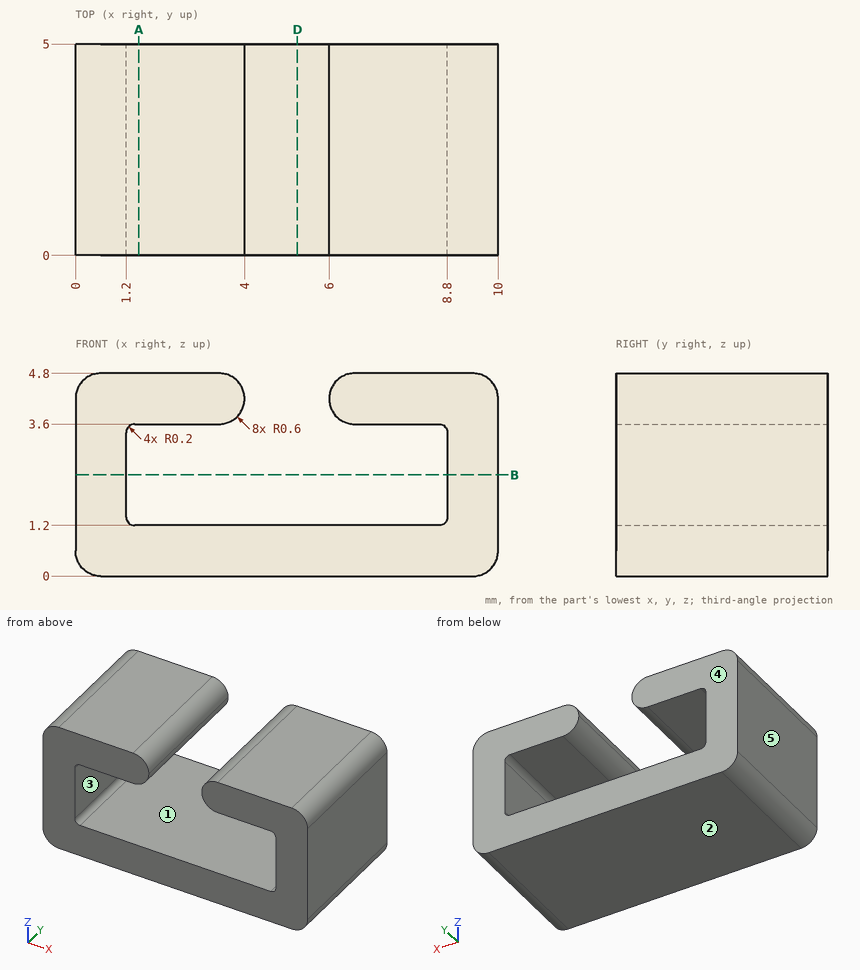
For this review, use the dimensioned drawing (mm, ordinates from the lowest corner) and the shaded views. A direction names the side the tool comes from. Round coordinates to 2 decimals unless told otherwise and drop trailing zeros. Write each loop counter-clockwise with the first axis right and the second up, starting at its lowest first coordinate (ties: lowest second). Pieces come first, ordered by that corner, then holes. Notation, with made-up numbers: (65.25, 46) -> (112.25, 46) arc R24 ccw to (112.25, 57) -> close; hole circle Ø3 at (38, 85). An arc over 180 degrees is marked (long way). Use CSV: the item, a comma, the result in double quotes.
(1) Draft analysis for pull direction X (two halves, no side actions). For the marked faces 3, 4 and 5, state which applies: +X half, -X half, draft (parallel to the pull), parting line (faces both ways), or undercut.
Computed values:
face 3,"undercut"
face 4,"draft"
face 5,"-X half"
(2) For the marked faces 1 and 2, list the 3-axis set-ups (+Z, -Z, +X, -X, +Y, -Y) from which the entire face can be reached by the end or side of a thin tool; tool diameter is ignored.
Computed values:
face 1,"+Y, -Y"
face 2,"-Z, +X, -X, +Y, -Y"
(3) Consider section D-D, the plane x = 5.25. Give the boundary of the cut face in (y, z), plus the area to 3 significant figures.
Computed values:
outline,"(0, 0) -> (5, 0) -> (5, 1.2) -> (0, 1.2) -> close"
area,"6.00 mm²"
(4) Clearance check with a flat-ended pin moving along its axis: P1, Ø1.5, axis at x = 5.5, y = 3, coming from the +Z side. State where the tip first meets the part, or that it passes through.
Computed values:
P1,"z = 4.69"
(5) Consider section B-B, the plane z = 2.4. Give the boundary of the cut face in (x, y).
Computed values:
outline,"(0, 0) -> (1.2, 0) -> (1.2, 5) -> (0, 5) -> close; (8.8, 0) -> (10, 0) -> (10, 5) -> (8.8, 5) -> close"
(6) To check wall thickness, follow L1, parallel to X at y = 1.75, z = 2.3; L2, parallel to Z at x = 2.5, y = 2.15; L3, parallel to X at y = 1.3, z = 4.2. State the ranges of each line that lie inside material, in increasing order. Write a range as [from, to].
Computed values:
L1,"[0, 1.2], [8.8, 10]"
L2,"[0, 1.2], [3.6, 4.8]"
L3,"[0, 4], [6, 10]"
(7) Consider section A-A, the plane x = 1.5. Give the boundary of the cut face in (y, z).
Computed values:
outline,"(0, 0) -> (5, 0) -> (5, 1.2) -> (0, 1.2) -> close; (0, 3.6) -> (5, 3.6) -> (5, 4.8) -> (0, 4.8) -> close"
